Study the drawing (mm; zero at the part's minimum x, y, z) and answer. A direction names the side the tool comes from. Coordinates: 2 decimals unless noted, no trailing zeros. Order: outer loops, then holes, each group sorted by start corner. A loop starts at its lowest first (then second) coordinate and runs counter-clockwise, first axis right, second up.
1. The part is cut by section A-A, the plane x = 21. Give the vertices of the cut face in (y, z), then the cut area to 3 significant figures.
2. A tool of negligible diameter and unlimited length cuts with its end or side. For the marked faces 4 and 5, from which of +Z, -Z, +X, -X, +Y, -Y can it reach the whole face along a straight path? Write none if from no direction.
3. Determine the mould class of the marked faces 1, 2 and 3 for opening direction X: +X half, -X half, draft (parallel to the pull), parting line (faces both ways), or undercut.
4. Flat-ended cylindrical pins translate along their axes: pin 1 Ø3 at (y, z) = (4, 3.5) entering from -X; pin 2 Ø13 at (x, y) = (21, 19.5) entering from -Z; pin 3 Ø12 at (x, y) = (16.5, 12.5) entering from +Z; pin 4 Ø1 at (x, z) = (9.5, 14.5) entering from +Y. Find the tip coordinate at first contact, or state that the pin passes through.
5. The part is cut by section B-B, the plane y = 19.5. Give the vertices of the cut face in (x, z), then the cut area to 3 significant figures.
6. Find the intervals of material crossed by probe 1 along X at (y, z) = (0.9, 14); probe 2 along Z at (x, y) = (28, 6); probe 3 along X at (y, z) = (22, 2.25), in increasing order.
7. The part is cut by section C-C, the plane z = 14. Give the vertices of the cut face in (x, y), then the cut area to 3 significant figures.
8. The part is cut by section D-D, the plane z = 2. Give the vertices of the cut face in (x, y) (1 decimal).
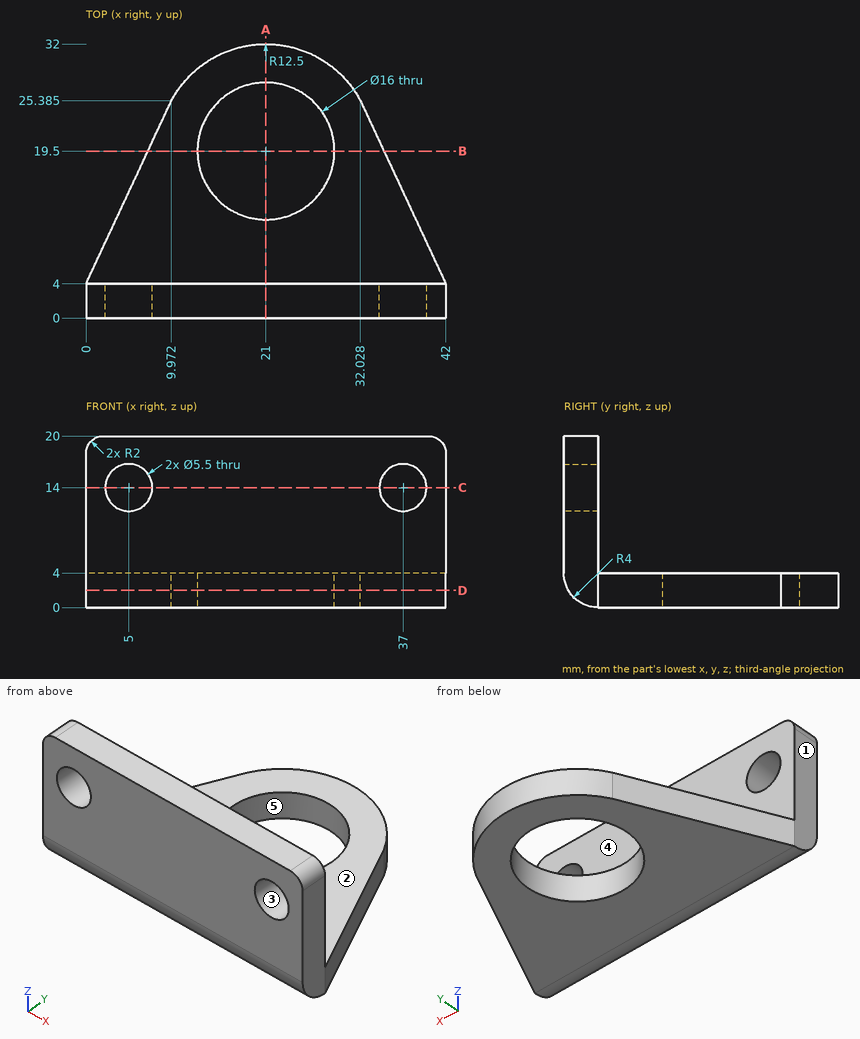
Geometry says:
1. outline: (0, 4) arc R4 ccw to (4, 0) - (11.5, 0) - (11.5, 4) - (4, 4) - (4, 20) - (0, 20) - close; (27.5, 0) - (32, 0) - (32, 4) - (27.5, 4) - close
1. area: 125 mm2
2. face 4: +Z, +X, -X, +Y
2. face 5: +Z, -Z
3. face 1: -X half
3. face 2: draft
3. face 3: undercut
4. pin 1: stops at x = 0
4. pin 2: passes through
4. pin 3: stops at z = 4
4. pin 4: stops at y = 4
5. outline: (7.23, 0) - (13, 0) - (13, 4) - (7.23, 4) - close; (29, 0) - (34.77, 0) - (34.77, 4) - (29, 4) - close
5. area: 46.2 mm2
6. probe 1: x = 0 to 2.25, 7.75 to 34.25, 39.75 to 42
6. probe 2: z = 0 to 4
6. probe 3: x = 8.39 to 13.4, 28.6 to 33.61
7. outline: (0, 0) - (2.25, 0) - (2.25, 4) - (0, 4) - close; (7.75, 0) - (34.25, 0) - (34.25, 4) - (7.75, 4) - close; (39.75, 0) - (42, 0) - (42, 4) - (39.75, 4) - close
7. area: 124 mm2
8. outline: (0, 0.5) - (42, 0.5) - (42, 4) - (32, 25.4) arc R12.5 ccw to (10, 25.4) - (0, 4) - close; hole circle Ø16 at (21, 19.5)
